Design review of the part built by this model. Coordinates are the model's own, in mm. Round coordinates to 2 decimals unless told otherwise and drop trailing zeros. Order: outer loops, then holes, each group sorted by start corner. A loop starts at its lowest first (then second) coordinate and runs counter-clockwise, first axis right, second up. Notation, with made-up numbers: M 32.25,-15.75 L 49.25,-15.75 A19 cw 49.25,-11.75 Z; hole C 56.25,-15.75 d7. An arc over 180 degrees is marked long. Write each question's results on one line, items separated by ' | '. Start each with the question number.
Item 1: Take a section at A-A, the plane x = 21.25. Write out the cut boundary in (y, z), plus the area to 3 significant figures.
Item 2: Wall thickness on line 1 (Y direction, x = 16.5, z = 0.75); line 2 (Y direction, x = 15.25, z = -1.55); line 3 (Z direction, x = 4, y = 2.25): over which ranges is each line inside the solid? List them lowest first. Write a range as [from, to].
Item 3: Clearance check with flat-ended pins moving along their axes: pin 1 (1.5 mm diameter, centred on y = 0.5, z = 1.5, fed in from -X); pin 2 (1 mm diameter, centred on x = 14, z = 2, fed in from -Y). State where each tip first meets the part, or that it passes through.
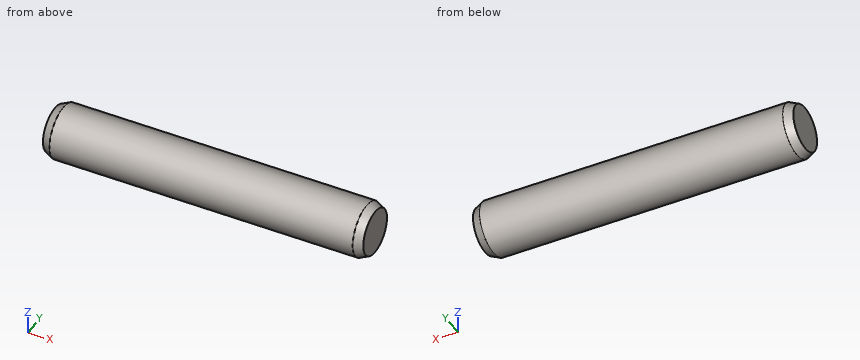
Autodesk Inventor part; units mm, degrees
ref_plane "YZ Plane" through (0, 0, 0) normal (1, 0, 0) x (0, 1, 0)
ref_plane "XZ Plane" through (0, 0, 0) normal (0, 1, 0) x (-1, 0, 0)
ref_plane "XY Plane" through (0, 0, 0) normal (0, 0, 1) x (1, 0, 0)
sketch "Эскиз" plane through (0, 0, 0) normal (1, 0, 0) x (0, 1, 0)
  circle A0 centre (0, 0) radius 2.5
  dimension "d1" = 5
extrude "Базовый элемент" add sketch "Эскиз" along normal blind 30
chamfer "Фаска1" distance 0.8 angle 25 1 edges at (0, -2.5, 0) measured on face at (20, 2.4919, -0.2012)
chamfer "Эскиз2" distance 0.8 angle 25 1 edges at (30, -2.5, 0) measured on face at (20.2667, 2.4919, -0.2012)
equation "\"d1\" = NND"
equation "\"d2\" = NLG"
equation "\"d8\" = PHH"
equation "\"d9\" = FAWI"
equation "\"d12\" = PHH"
equation "\"d4\" = PHH"
equation "\"d5\" = FAWI"
equation "\"d11\" = PHH"
equation "\"NND\" = 5"
equation "\"NLG\" = 30"
equation "\"PHH\" = 0.8"
equation "\"FAWI\" = 25deg"
equation "\"KAH\" = 0"
properties part number "Штифт 2.5x30 ГОСТ 3128-70" material "Сталь, мягкая"
Results list:
1) outline: C 0,0 d5 | area: 19.6 mm²
2) line 1: [-2.38, 2.38] | line 2: [-1.96, 1.96] | line 3: [-1.09, 1.09]
3) pin 1: x = 0 | pin 2: y = -2
